```python
from build123d import *

# Parameters (mm, degrees)
F0_R     = 6.75
F1_DEPTH = 1.5
F2_W     = 4
F2_H     = 4
F3_DEPTH = 6.5
F5_W     = 1
F5_H     = 6.2726680437
F6_DEPTH = 25
F7_R     = 1.99999
F8_R     = 1


# Not quite as in the source:
# - a fillet or chamfer is up to 0.001 mm smaller than in the source, because OpenCascade refuses the exact size


with BuildPart() as f1:
    # F0 (on Top) → F1 (new body)
    with BuildSketch(Plane.XY):
        Circle(F0_R)
    extrude(amount=F1_DEPTH)

    # F2 (on face) → F3 (join)
    with BuildSketch(Plane.XY.offset(1.5)):
        Rectangle(F2_W, F2_H)
    extrude(amount=F3_DEPTH)

    # F5 (on face) → F6 (cut)
    with BuildSketch(Plane.XZ.offset(2)):
        with Locations((0, 4.8636659781)):
            Rectangle(F5_W, F5_H)
    extrude(amount=-F6_DEPTH, mode=Mode.SUBTRACT)

    # F7 (radius 2 in the source; OpenCascade refuses exactly that, so slightly less here)
    f7_edges = [f1.edges().sort_by_distance(p)[0] for p in [
        (2, -2, 4.75),
        (2, 2, 4.75),
        (-2, 2, 4.75),
        (-2, -2, 4.75),
    ]]
    fillet(f7_edges, radius=F7_R)

    # F8
    f8_edges = [f1.edges().sort_by_distance(p)[0] for p in [
        (1.581139, 1.224752, 8),
        (-1.581139, 1.224752, 8),
    ]]
    fillet(f8_edges, radius=F8_R)


solid = f1.part
```
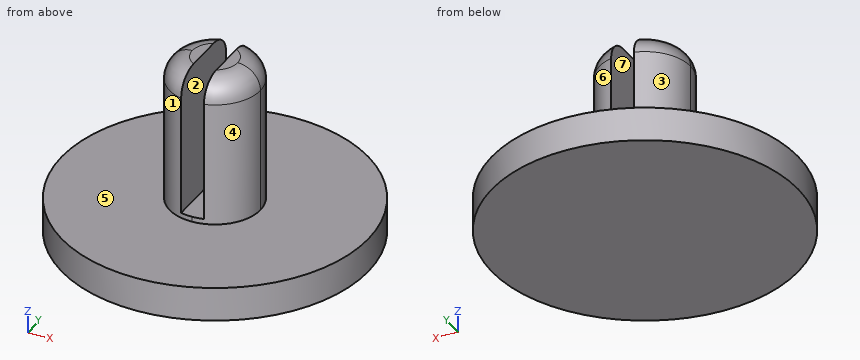
Verification items for the finished model (mm, model axes). Face numbers are marked on the shaded views. A direction names the side the tool comes from. Give positions to 0.01 mm unless a question says otherwise; leave off trailing zeros. Order: outer loops, then holes, each group sorted by start corner. A loop starts at its lowest first (then second) coordinate and runs counter-clockwise, first axis right, second up. Notation, with made-up numbers: (2.25, 89.5) -> (55.25, 89.5) arc R24 ccw to (55.25, 126.5) -> close; hole circle Ø6 at (-38.5, 15.25). An arc over 180 degrees is marked (long way). Use a Markdown table: item, result.
1) Section check C-C, the plane y = 5. Record the boundary of the cut face in (x, z), then the cut area to 3 significant figures.
Results:
| item | result |
|---|---|
| outline | (-4.53, 0) -> (4.53, 0) -> (4.53, 1.5) -> (-4.53, 1.5) -> close |
| area | 13.6 mm² |
2) Tool access check on the marked faces 1, 2, 3 and 4. Record the directions out of +Z, -Z, +X, -X, +Y, -Y that give a thin tool (end or side, any length) a straight path to the whole face; none if there is none.
Results:
| item | result |
|---|---|
| face 1 | +Z, -X, -Y |
| face 2 | +Z, +Y, -Y |
| face 3 | +Z, -X, +Y |
| face 4 | +Z, +X, -Y |
3) Material ranges on probe 1 along Z at (x, y) = (1.75, -5.5); probe 2 along X at (y, z) = (0.5, 3.25); probe 3 along X at (y, z) = (-1, 7.5), recorded low to high.
Results:
| item | result |
|---|---|
| probe 1 | 0 to 1.5 |
| probe 2 | -1.94 to -0.5, 0.5 to 1.94 |
| probe 3 | -1.58 to -0.5, 0.5 to 1.58 |
4) Mould release check, pull along X, two halves, no side actions. Record for the marked faces 5, 6 and 7: pulls with the +X half, pulls with the -X half, needs draft (parallel to the pull), parting line crosses it, or undercut.
Results:
| item | result |
|---|---|
| face 5 | needs draft |
| face 6 | pulls with the +X half |
| face 7 | undercut |
5) Depth check by flat-ended pin: pin 1 Ø0.5 at (x, y) = (0, 0) entering from +Z; pin 2 Ø1.5 at (x, y) = (0.5, 1.5) entering from -Z; pin 3 Ø3 at (y, z) = (0, 4.5) entering from -X; pin 4 Ø1.9 at (y, z) = (-0.5, 4) entering from +X. Enter the tip coordinate at first touch or a pass-through.
Results:
| item | result |
|---|---|
| pin 1 | z = 1.73 |
| pin 2 | z = 0 |
| pin 3 | x = -2 |
| pin 4 | x = 2 |
6) Section check B-B, the plane x = -5.75. Record the boundary of the cut face in (y, z), then the cut area to 3 significant figures.
Results:
| item | result |
|---|---|
| outline | (-3.54, 0) -> (3.54, 0) -> (3.54, 1.5) -> (-3.54, 1.5) -> close |
| area | 10.6 mm² |
